```python
from build123d import *

# Parameters (mm, degrees)
F1_DEPTH = 29
F2_W     = 36
F2_H     = 11
F3_DEPTH = 116.001
F4_R     = 3
F5_W     = 19
F5_H     = 13
F6_DEPTH = 27.001


with BuildPart() as f1:
    # F0 (on Front) → F1 (new body, symmetric)
    with BuildSketch(Plane.XZ):
        with BuildLine():
            Line((-52.5, 0), (0, 0))
            Line((0, 0), (52.5, 0))
            Line((52.5, 0), (52.5, 9))
            Line((52.5, 9), (63.5, 9))
            ThreePointArc((63.5, 9), (55.006097, 29.506097), (34.5, 38))
            Line((34.5, 38), (0, 38))
            Line((0, 38), (-34.5, 38))
            ThreePointArc((-34.5, 38), (-55.006097, 29.506097), (-63.5, 9))
            Line((-63.5, 9), (-52.5, 9))
            Line((-52.5, 9), (-52.5, 0))
        make_face()
    extrude(amount=F1_DEPTH, both=True)

    # F2 (on face) → F3 (cut, through all)
    with BuildSketch(Plane.YZ.offset(52.5)):
        with Locations((0, 32.5)):
            Rectangle(F2_W, F2_H)
    extrude(amount=-F3_DEPTH, mode=Mode.SUBTRACT)

    # F4
    f4_edges = [f1.edges().sort_by_distance(p)[0] for p in [
        (0, 29, 38),
        (0, -29, 38),
    ]]
    fillet(f4_edges, radius=F4_R)

    # F5 (on face) → F6 (cut, through all)
    with BuildSketch(Plane.XY.offset(27)):
        with BuildLine():
            ThreePointArc((-38.5, 6.5), (-45, 0), (-38.5, -6.5))
            Line((-38.5, -6.5), (-38.5, 6.5))
        make_face()
        with Locations((-29, 0)):
            Rectangle(F5_W, F5_H)
        with BuildLine():
            Line((-19.5, 6.5), (-19.5, -6.5))
            ThreePointArc((-19.5, -6.5), (-13, 0), (-19.5, 6.5))
        make_face()
        with BuildLine():
            ThreePointArc((38.5, -6.5), (45, 0), (38.5, 6.5))
            Line((38.5, 6.5), (19.5, 6.5))
            ThreePointArc((19.5, 6.5), (13, 0), (19.5, -6.5))
            Line((19.5, -6.5), (38.5, -6.5))
        make_face()
    extrude(amount=-F6_DEPTH, mode=Mode.SUBTRACT)


solid = f1.part
```
Geometry check sheet. Reference: the model listing, model coordinates, mm. A direction names the side the tool comes from. Give positions to 0.01 mm unless a question says otherwise; leave off trailing zeros. Order: outer loops, then holes, each group sorted by start corner. A loop starts at its lowest first (then second) coordinate and runs counter-clockwise, first axis right, second up. Notation, with made-up numbers: (-4, 69) -> (27, 69) arc R22 cw to (27, 102) -> close; hole circle Ø2 at (72.25, -12). An arc over 180 degrees is marked (long way). Write each question's results on one line, items separated by ' | '. Start each with the question number.
(1) Sectioned sample at B-B (y = 2.5). Enter the section's corners in (x, z), plus the area to 3 significant figures.
(2) Access from +Z, -Z, +X, -X, +Y, -Y to the whole of each face (thin tool, end or side, straight path). Record for faces 1 (the face through (45, 0, 14)), 2 (the face through (58, 0, 9)), 3 (the face through (-2, 18, 32)), 4 (the face through (-1, -29, 18)), 5 (the face through (-58, 0, 9)).
(3) Sectioned sample at D-D (x = 0.5). Enter the section's corners in (y, z), plus the area to 3 significant figures.
(4) Scan lines: line 1 (Y direction, x = 36, z = 29); line 2 (X direction, y = 1.5, z = 18.5); line 3 (Y direction, x = -36, z = 2.5). Record each from-to range of solid material in increasing order.
(5) Sectioned sample at C-C (y = 10.5). Enter the section's corners in (x, z), plus the area to 3 significant figures.
(6) Mould release check, pull along X, two halves, no side actions. Record for faces 6 (the face through (-2, -18, 32)), 7 (the face through (-60.65, -0.36, 21.54)), 8 (the face through (52.5, 0, 4)), 9 (the face through (-29, -6.5, 14)): pulls with the +X half, pulls with the -X half, needs draft (parallel to the pull), parting line crosses it, or undercut.
(7) Gauge pin test, flat ends, axial feed: P1, Ø5, axis at x = 50.5, y = 0, coming from the -Z side; P2, Ø4.5, axis at y = 7.5, z = 4.5, coming from the -X side; P3, Ø4, axis at y = -15.5, z = 11.5, coming from the -X side; P4, Ø5, axis at y = 16.5, z = 15.5, coming from the -X side. Record the tip position at first contact, or that the pin passes through.
(8) Sectioned sample at A-A (x = -33). Enter the section's corners in (y, z).
Answer below:
1) outline: (-63.5, 9) -> (-52.5, 9) -> (-52.5, 0) -> (-44.5, 0) -> (-44.5, 27) -> (-57.24, 27) arc R29 ccw to start; (-13.5, 0) -> (13.5, 0) -> (13.5, 27) -> (-13.5, 27) -> close; (44.5, 0) -> (52.5, 0) -> (52.5, 9) -> (63.5, 9) arc R29 ccw to (52.5, 31.74) -> (52.5, 27) -> (44.5, 27) -> close | area: 1,500 mm2
2) face 1: +Z, -Z | face 2: -Z, +X, +Y, -Y | face 3: +Z, -X | face 4: +Z, -Z, +X, -X, -Y | face 5: -Z, -X, +Y, -Y
3) outline: (-29, 0) -> (29, 0) -> (29, 35) arc R3 ccw to (26, 38) -> (18, 38) -> (18, 27) -> (-18, 27) -> (-18, 38) -> (-26, 38) arc R3 ccw to (-29, 35) -> close | area: 1,800 mm2
4) line 1: -29 to -18, 18 to 29 | line 2: -61.9 to -44.82, -13.18 to 13.18, 44.82 to 61.9 | line 3: -29 to -6.5, 6.5 to 29
5) outline: (-63.5, 9) -> (-52.5, 9) -> (-52.5, 0) -> (52.5, 0) -> (52.5, 9) -> (63.5, 9) arc R29 ccw to (52.5, 31.74) -> (52.5, 27) -> (-57.24, 27) arc R29 ccw to start | area: 3,170 mm2
6) face 6: needs draft | face 7: pulls with the -X half | face 8: pulls with the +X half | face 9: undercut
7) P1: z = 0 | P2: x = -52.5 | P3: x = -63.5 | P4: x = -63.22
8) outline: (-29, 0) -> (-6.5, 0) -> (-6.5, 27) -> (-18, 27) -> (-18, 38) -> (-26, 38) arc R3 ccw to (-29, 35) -> close; (6.5, 0) -> (29, 0) -> (29, 35) arc R3 ccw to (26, 38) -> (18, 38) -> (18, 27) -> (6.5, 27) -> close
